Design review of the part built by this model. Coordinates are the model's own, in mm. Face numbers are marked on the shaded views. A direction names the side the tool comes from. Coordinates: 2 decimals unless noted, no trailing zeros. Order: outer loops, then holes, each group sorted by start corner. A loop starts at its lowest first (then second) coordinate and runs counter-clockwise, first axis right, second up. Notation, with made-up numbers: M 78.25,86 L 101.25,86 A20 cw 101.25,124 Z; hole C 37.25,25.25 d9. An arc over 180 degrees is marked long. Answer as a JSON object with one key per item and string values.
from build123d import *
from build123d.topology import SkipClean

# Parameters (mm, degrees)
SKETCH1_R               = 38.1
BOSS_EXTRUDE1_DEPTH     = 76.2
SHELL2_T                = 3.175
SKETCH2_W               = 3
SKETCH2_H               = 82.55
BOSS_EXTRUDE2_DEPTH     = 4
CUT_EXTRUDE1_DEPTH      = 99.527366122
CUT_EXTRUDE1_DEPTH_BACK = 99.527366122
SKETCH3_R               = 61.906276858
SKETCH3_R_2             = 41.275


with BuildPart() as part:
    # Sketch1 → Boss-Extrude1 (new body)
    with BuildSketch(Plane(origin=(0, 0, 0), x_dir=(1, 0, 0), z_dir=(0, 1, 0))):
        with Locations(Location((0, 0, 0), (0, 0, 90))):
            Circle(SKETCH1_R)
    extrude(amount=BOSS_EXTRUDE1_DEPTH)

    # Shell2
    shell2_openings = [part.faces().sort_by_distance(p)[0] for p in [
        (0, 76.2, 0),
    ]]
    offset(amount=SHELL2_T, openings=shell2_openings, kind=Kind.INTERSECTION)

    # Sketch2 → Boss-Extrude2 (add)
    with BuildSketch(Plane(origin=(0, -3.175, 0), x_dir=(-1, 0, 0), z_dir=(0, -1, 0))):
        Rectangle(SKETCH2_W, SKETCH2_H)
        Polygon((-23.047310797, -34.273854321), (25.47436178, 32.510498564), (23.047310797, 34.273854321), (-25.47436178, -32.510498564), align=None)
        Polygon((-38.791332219, -14.181261217), (39.718383202, 11.328091668), (38.791332219, 14.181261217), (-39.718383202, -11.328091668), align=None)
        Polygon((-39.718383202, 11.328091668), (38.791332219, -14.181261217), (39.718383202, -11.328091668), (-38.791332219, 14.181261217), align=None)
        Polygon((-25.47436178, 32.510498564), (23.047310797, -34.273854321), (25.47436178, -32.510498564), (-23.047310797, 34.273854321), align=None)
    extrude(amount=BOSS_EXTRUDE2_DEPTH)

    # Sketch3 → Cut-Extrude1 (cut, two sides: drawn at the far end of the back side and taken through both)
    with SkipClean():  # the faces are left unmerged after this step: merging them gives an invalid solid
        with BuildSketch(Plane.XZ.offset(3.175).offset(-CUT_EXTRUDE1_DEPTH_BACK)):
            Circle(SKETCH3_R)
            with Locations(Location((0, 0, 0), (0, 0, 272.082679548))):
                Circle(SKETCH3_R_2, mode=Mode.SUBTRACT)
        extrude(amount=CUT_EXTRUDE1_DEPTH + CUT_EXTRUDE1_DEPTH_BACK, mode=Mode.SUBTRACT)


solid = part.part
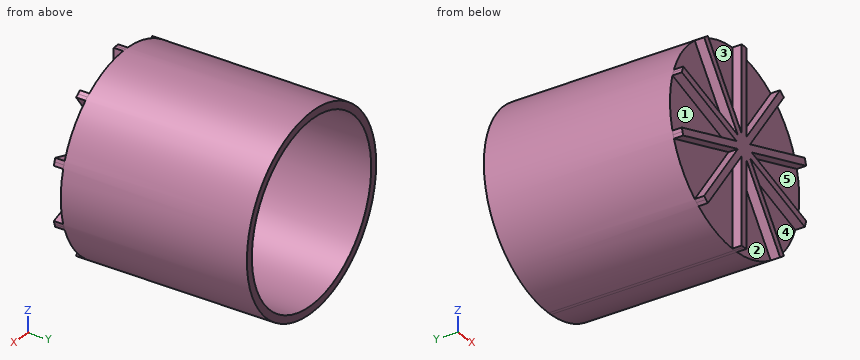
1) Add section D-D (z = -26). State the section outline as (x, y) points (3 decimals), and give its area (3 significant figures).
Taken from the geometry:
{"outline": "M -32.057,-3.175 L -20.744,-3.175 L -20.744,-7.175 L -17.036,-7.175 L -17.036,-3.175 L -1.5,-3.175 L -1.5,-7.175 L 1.5,-7.175 L 1.5,-3.175 L 17.036,-3.175 L 17.036,-7.175 L 20.744,-7.175 L 20.744,-3.175 L 32.057,-3.175 L 32.057,76.2 L 27.85,76.2 L 27.85,0 L -27.85,0 L -27.85,76.2 L -32.057,76.2 Z", "area": "886 mm2"}
2) Add section C-C (x = 6.5). State the section outline as (y, z) points (3 decimals), and give its area (3 significant figures).
Taken from the geometry:
{"outline": "M -7.175,-11.498 L -3.175,-11.498 L -3.175,-40.76 L 76.2,-40.76 L 76.2,-37.541 L 0,-37.541 L 0,37.541 L 76.2,37.541 L 76.2,40.76 L -3.175,40.76 L -3.175,11.498 L -7.175,11.498 L -7.175,6.395 L -3.175,6.395 L -3.175,3.689 L -7.175,3.689 L -7.175,0.535 L -3.175,0.535 L -3.175,-0.535 L -7.175,-0.535 L -7.175,-3.689 L -3.175,-3.689 L -3.175,-6.395 L -7.175,-6.395 Z", "area": "815 mm2"}
3) Insertion check: pin 1 Ø3 at (y, z) = (-5.5, -28) entering from -X; pin 2 Ø4.5 at (y, z) = (-6, -17) entering from +X; pin 3 Ø10 at (x, y) = (18.5, 2) entering from +Z. Each pin has a flat end and moves straight along its axis. Give the tip position at first contact, or say it passes through.
Taken from the geometry:
{"pin 1": "stops at x = -23.29", "pin 2": "stops at x = 15.84", "pin 3": "stops at z = 39"}
4) Add section A-A (y = 1.5). State the section outline as (x, z) points (3 decimals), and give its area (3 significant figures).
Taken from the geometry:
{"outline": "C 0,0 d82.55; hole C 0,0 d76.2", "area": "792 mm2"}
5) Tool access review of the marked faces 3, 4 and 5: name each direction out of +Z, -Z, +X, -X, +Y, -Y from which nothing blocks a thin tool from reaching the whole face with its end or side.
Taken from the geometry:
{"face 3": "+Z, -Y", "face 4": "-Y", "face 5": "+X, -Y"}
6) Add section B-B (z = 31). State the section outline as (x, y) points (3 decimals), and give its area (3 significant figures).
Taken from the geometry:
{"outline": "M -27.251,-3.175 L -24.377,-3.175 L -24.377,-7.175 L -20.669,-7.175 L -20.669,-3.175 L -1.5,-3.175 L -1.5,-7.175 L 1.5,-7.175 L 1.5,-3.175 L 20.669,-3.175 L 20.669,-7.175 L 24.377,-7.175 L 24.377,-3.175 L 27.251,-3.175 L 27.251,76.2 L 22.15,76.2 L 22.15,0 L -22.15,0 L -22.15,76.2 L -27.251,76.2 Z", "area": "992 mm2"}
7) To check wall thickness, follow L1, parallel to X at y = 33.5, z = 0 (3 decimals); L2, parallel to Y at x = -23, z = -16.5 (3 decimals); L3, parallel to Y at x = 3, z = -5 (3 decimals). State the ranges of each line that lie inside material, in increasing order.
Taken from the geometry:
{"L1": "x = -41.275 to -38.1, 38.1 to 41.275", "L2": "y = -3.175 to 0", "L3": "y = -7.175 to 0"}
8) Mouldability with a two-part tool opening along Z and no side actions: class the marked faces 1 and 2 as released by +Z, released by -Z, zero draft, split by the parting line, or undercut.
Taken from the geometry:
{"face 1": "undercut", "face 2": "zero draft"}
